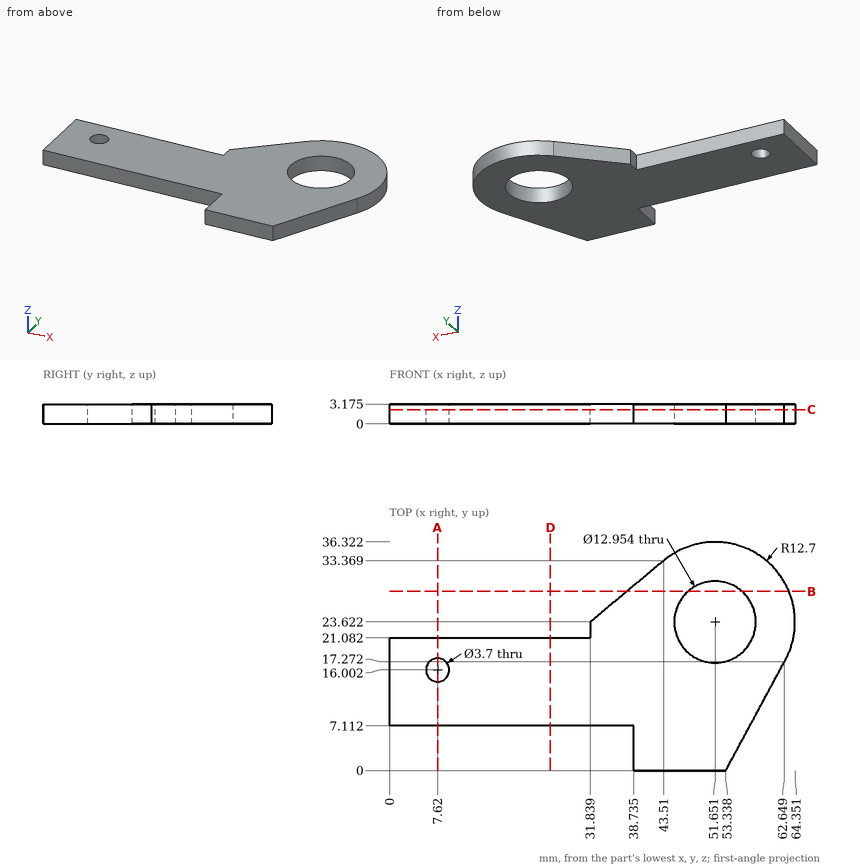
Geometry: see drawing. Coordinates: mm, zero at the bounding-box minimum. Coordinates: 2 decimals unless noted, no trailing zeros. Order: outer loops, then holes, each group sorted by start corner. A loop starts at its lowest first (then second) coordinate and runs counter-clockwise, first axis right, second up. Notation, with made-up numbers: (44.5, 37.5) - (73.5, 37.5) arc R26 ccw to (73.5, 66.5) - close; hole circle Ø3 at (57, 8.25). An arc over 180 degrees is marked (long way). Write each question's results on one line, items separated by ' | '.
(1) Line query: line 1 (Y direction, x = 7.5, z = 1.6) (1 decimal); line 2 (Y direction, x = 7.62, z = 1.3); line 3 (Y direction, x = 24, z = 2.3). Output: solid intervals per line, ascending. Write a range as [from, to].
Values found:
line 1: y = [7.1, 14.2], [17.8, 21.1] | line 2: y = [7.11, 14.15], [17.85, 21.08] | line 3: y = [7.11, 21.08]
(2) Section query B-B, the plane y = 28.5. Return the cut outline in (x, z) (1 decimal).
Values found:
outline: (37.7, 0) - (47.4, 0) - (47.4, 3.2) - (37.7, 3.2) - close; (55.9, 0) - (63.4, 0) - (63.4, 3.2) - (55.9, 3.2) - close
(3) Section query D-D, the plane x = 25.5. Return the cut outline in (y, z) (1 decimal).
Values found:
outline: (7.1, 0) - (21.1, 0) - (21.1, 3.2) - (7.1, 3.2) - close
(4) First-contact query: pin 1 Ø0.8 at (y, z) = (22, 1.5) entering from -X. Flat tip, straight axial feed; report the tip coordinate or a pass-through.
Values found:
pin 1: stops at x = 31.84
(5) Section query A-A, the plane x = 7.62. Return the cut outline in (y, z) (1 decimal), plus the area to 3 significant figures.
Values found:
outline: (7.1, 0) - (14.2, 0) - (14.2, 3.2) - (7.1, 3.2) - close; (17.9, 0) - (21.1, 0) - (21.1, 3.2) - (17.9, 3.2) - close | area: 32.6 mm²
(6) Section query C-C, the plane z = 2.3. Count the separate pieces of the cut face and the enclosed holes in it, plus the area to 3 significant figures.
Values found:
separate pieces: 1 | enclosed holes: 2 | area: 1,190 mm²
